Autodesk Inventor part; units mm, degrees
ref_plane "YZ Plane" through (0, 0, 0) normal (1, 0, 0) x (0, 1, 0)
ref_plane "XZ Plane" through (0, 0, 0) normal (0, 1, 0) x (-1, 0, 0)
ref_plane "XY Plane" through (0, 0, 0) normal (0, 0, 1) x (1, 0, 0)
sketch "Sketch1" plane through (0, 0, 0) normal (0, 1, 0) x (-1, 0, 0)
  circle A0 centre (0, 0) radius 2
  dimension "d0" = 4
extrude "Extrusion1" add sketch "Sketch1" along normal blind 2
sketch "Sketch2" plane through (0, 0, 0) normal (0, -1, 0) x (1, 0, 0)
  circle A0 centre (0, 0) radius 1.25
  dimension "d3" = 2.5
extrude "Extrusion2" add sketch "Sketch2" along normal blind 12
thread "Thread1"
sketch "Sketch3" plane through (0, 2, 0) normal (0, 1, 0) x (1, 0, 0)
  circle A0 centre (0, 0) radius 1.25
  line L0 (0.0005, 1.4434) -> (1.2502, 0.7213)
  line L1 (1.2502, 0.7213) -> (1.2498, -0.7221)
  line L2 (1.2498, -0.7221) -> (-0.0005, -1.4434)
  line L3 (-0.0005, -1.4434) -> (-1.2502, -0.7213)
  line L4 (-1.2502, -0.7213) -> (-1.2498, 0.7221)
  line L5 (-1.2498, 0.7221) -> (0.0005, 1.4434)
  point P0 (-0.6247, 1.0827)
extrude "Extrusion3" cut sketch "Sketch3" against normal blind 1
properties part number "screwM2-5"
The listing builds one solid part. Answer for the finished solid, in the listing's coordinates (mm). A direction names the side the tool comes from. Round coordinates to 2 decimals unless told otherwise and drop trailing zeros. Order: outer loops, then holes, each group sorted by start corner. A loop starts at its lowest first (then second) coordinate and runs counter-clockwise, first axis right, second up. Notation, with made-up numbers: M 73.5,59.25 L 121.5,59.25 A24 ccw 121.5,80.25 Z; hole C -32,86 d1. An arc over 180 degrees is marked long. Answer in a Markdown table with one row per item. Add a question column.
1) The part is cut by section B-B on x = 0.95. Determine the outline of the cut face in (y, z).
2) The part is cut by section D-D on x = 1.5. Determine the outline of the cut face in (y, z), plus the area to 3 significant figures.
3) Consider line 1 along Y through (x, z) = (0.7, 0.75); line 2 along Y through (x, z) = (-1.6, -0.15); line 3 along Z through (x, y) = (0.9, 1.5). Determine where each line is inside the solid, lowest interval first. Write a range as from..to.
4) Flat-ended cylindrical pins translate along their axes: pin 1 Ø1 at (x, y) = (0, -5) entering from +Z; pin 2 Ø0.8 at (x, z) = (0, -0.5) entering from +Y; pin 3 Ø2 at (x, y) = (0.5, -10) entering from -Z; pin 4 Ø2 at (x, z) = (-1.5, 0.5) entering from -Y. Find the tip coordinate at first contact, or state that the pin passes through.
5) Determine the mould class of faces 1 (the face through (0, 1, 2)), 2 (the face through (0.617, 1.507, -1.087)), 3 (the face through (-1, 0, 1)) for opening direction Z: pulls with the +Z half, pulls with the -Z half, needs draft (parallel to the pull), parting line crosses it, or undercut.
6) Which of the six approach directions +Z, -Z, +X, -X, +Y, -Y give full straight-line access (tool end or side, diameter ignored) to faces 4 (the face through (-0.617, 1.507, 1.087)), 5 (the face through (-0.27, -5.92, 1.22)), 6 (the face through (0, -12, 0))?
7) The part is cut by section A-A on z = 0. Determine the outline of the cut face in (x, y).
8) The part is cut by section C-C on y = -7.5. Determine the outline of the cut face in (x, z), plus the area to 3 significant figures.
Findings below:
| question | item | result |
|---|---|---|
| 1 | outline | M -12,-0.81 L 0,-0.81 L 0,-1.76 L 2,-1.76 L 2,-0.89 L 1,-0.89 L 1,0.9 L 2,0.9 L 2,1.76 L 0,1.76 L 0,0.81 L -12,0.81 Z |
| 2 | outline | M 0,-1.32 L 2,-1.32 L 2,1.32 L 0,1.32 Z |
| 2 | area | 5.29 mm² |
| 3 | line 1 | y = -12..1 |
| 3 | line 2 | y = 0..2 |
| 3 | line 3 | z = -1.79..-0.92, 0.92..1.79 |
| 4 | pin 1 | stops at z = 1.25 |
| 4 | pin 2 | stops at y = 1 |
| 4 | pin 3 | stops at z = -1.25 |
| 4 | pin 4 | stops at y = -12 |
| 5 | face 1 | parting line crosses it |
| 5 | face 2 | undercut |
| 5 | face 3 | needs draft |
| 6 | face 4 | +Y |
| 6 | face 5 | -Y |
| 6 | face 6 | +Z, -Z, +X, -X, -Y |
| 7 | outline | M -2,0 L -1.25,0 L -1.25,-12 L 1.25,-12 L 1.25,0 L 2,0 L 2,2 L 1.25,2 L 1.25,1 L -1.25,1 L -1.25,2 L -2,2 Z |
| 8 | outline | C 0,0 d2.5 |
| 8 | area | 4.91 mm² |
